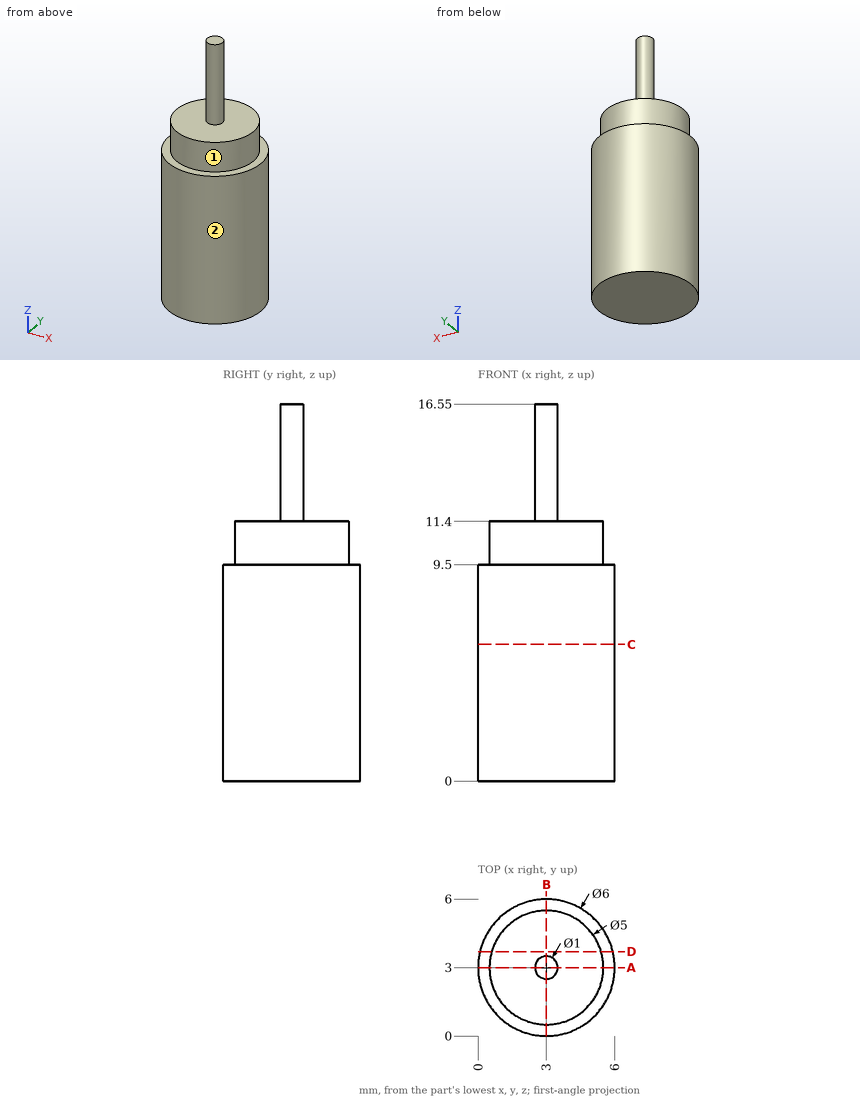
Print and shaded views of the part. All mm, measured from the part's lowest x, y and z. A direction names the side the tool comes from. Coordinates: 2 decimals unless noted, no trailing zeros. Order: outer loops, then holes, each group sorted by start corner. A loop starts at its lowest first (then second) coordinate and runs counter-clockwise, first axis right, second up.
(1) Probe L1, parallel to Z at x = 5.4, y = 4.25; L2, parallel to Z at x = 2.55, y = 4.15; L3, parallel to Y at x = 2.9, z = 2.75. List the from-to ranges inside material, lowest first.
Check sheet entries:
L1: z = 0 to 9.5
L2: z = 0 to 11.4
L3: y = 0 to 6
(2) Slice it at D-D, the plane y = 3.7. Write the cut outline in (x, z), and give its area (3 significant figures).
Check sheet entries:
outline: (0.08, 0) - (5.92, 0) - (5.92, 9.5) - (5.4, 9.5) - (5.4, 11.4) - (0.6, 11.4) - (0.6, 9.5) - (0.08, 9.5) - close
area: 64.5 mm2
(3) Tool access for the marked faces 1 and 2: list every direction of +Z, -Z, +X, -X, +Y, -Y with a clear straight run to the whole face (end or side of a thin tool).
Check sheet entries:
face 1: +Z
face 2: +Z, -Z
(4) Slice it at A-A, the plane y = 3. Write the cut outline in (x, z).
Check sheet entries:
outline: (0, 0) - (6, 0) - (6, 9.5) - (5.5, 9.5) - (5.5, 11.4) - (3.5, 11.4) - (3.5, 16.55) - (2.5, 16.55) - (2.5, 11.4) - (0.5, 11.4) - (0.5, 9.5) - (0, 9.5) - close
(5) Slice it at C-C, the plane z = 6. Write the cut outline in (x, y).
Check sheet entries:
outline: circle Ø6 at (3, 3)
(6) Pin check, flat tips, straight feed: pin 1 Ø3 at (y, z) = (4.5, 15) entering from +X; pin 2 Ø3 at (y, z) = (4, 12.5) entering from -X; pin 3 Ø1.5 at (x, y) = (4, 2.5) entering from +Z; pin 4 Ø1 at (y, z) = (1, 6.5) entering from -X. Stop position of each tip, or through.
Check sheet entries:
pin 1: stops at x = 3.5
pin 2: stops at x = 0.5
pin 3: stops at z = 16.55
pin 4: stops at x = 0.4
